from build123d import *

# Parameters (mm, degrees)
SKETCH1_R                = 2.5
BOSS_EXTRUDE1_DEPTH      = 4
CONVERT_SOLID1_OUTLINE_R = 2.5
CONVERT_SOLID1_DEPTH     = 2.5
EDGE_FLANGE1_DEPTH       = 20
EDGE_FLANGE1_BEND_DEPTH  = 20
EDGE_FLANGE2_DEPTH       = 20
EDGE_FLANGE2_BEND_DEPTH  = 20
SKETCH14_R               = 2.5
CUT_EXTRUDE1_DEPTH       = 4


# Read off the part's stored shape, not the designer's step: Convert-Solid1
# Sheet-metal steps are written as plain solids
with BuildPart() as part:
    # Sketch1 → Boss-Extrude1 (new body)
    with BuildSketch(Plane.XY):
        with BuildLine():
            Line((-474.195090562, 127.525252525), (-477.445756062, 127.525252525))
            ThreePointArc((-477.445756062, 127.525252525), (-484.91471638, 109.01150893), (-490.83715139, 89.946650322))
            Line((-490.83715139, 89.946650322), (-520.264617773, 89.946650322))
            Line((-520.264617773, 89.946650322), (-520.264617773, 69.946650322))
            Line((-520.264617773, 69.946650322), (-495.264617773, 69.946650322))
            ThreePointArc((-495.264617773, 69.946650322), (-499, 27.525252525), (-495.264617773, -14.896145272))
            Line((-495.264617773, -14.896145272), (-520.264617773, -14.896145272))
            Line((-520.264617773, -14.896145272), (-520.264617773, -34.896145272))
            Line((-520.264617773, -34.896145272), (-490.83715139, -34.896145272))
            ThreePointArc((-490.83715139, -34.896145272), (-484.91471638, -53.961003879), (-477.445756062, -72.474747475))
            Line((-477.445756062, -72.474747475), (-474.195090562, -72.474747475))
            ThreePointArc((-474.195090562, -72.474747475), (-470.012418883, -70.21432), (-469.611597595, -65.476850524))
            ThreePointArc((-469.611597595, -65.476850524), (-489, 27.525252525), (-469.611597595, 120.527355575))
            ThreePointArc((-469.611597595, 120.527355575), (-470.012418883, 125.264825051), (-474.195090562, 127.525252525))
        make_face()
        with Locations(Location((-488.148813177, 79.946650322, 0), (0, 0, 180))):
            Circle(SKETCH1_R, mode=Mode.SUBTRACT)
        with Locations((-494, 27.525252525)):
            Circle(SKETCH1_R, mode=Mode.SUBTRACT)
        with Locations((-488.148813177, -24.896145272)):
            Circle(SKETCH1_R, mode=Mode.SUBTRACT)
        with Locations((-476.297445473, -62.474747475)):
            Circle(SKETCH1_R, mode=Mode.SUBTRACT)
        with Locations(Location((-476.297445473, 117.525252525, 0), (0, 0, 180))):
            Circle(SKETCH1_R, mode=Mode.SUBTRACT)
    extrude(amount=BOSS_EXTRUDE1_DEPTH)

    # Convert-Solid1 outline → Convert-Solid1 (cut)
    with BuildSketch(Plane.XY):
        with BuildLine():
            ThreePointArc((-490.83715139, -34.896145272), (-484.91471638, -53.961003879), (-477.445756062, -72.474747475))
            Line((-477.445756062, -72.474747475), (-474.195090562, -72.474747475))
            ThreePointArc((-474.195090562, -72.474747475), (-470.012418883, -70.21432), (-469.611597595, -65.476850524))
            ThreePointArc((-469.611597595, -65.476850524), (-489, 27.525252525), (-469.611597595, 120.527355575))
            ThreePointArc((-469.611597595, 120.527355575), (-470.012418883, 125.264825051), (-474.195090562, 127.525252525))
            Line((-474.195090562, 127.525252525), (-477.445756062, 127.525252525))
            ThreePointArc((-477.445756062, 127.525252525), (-484.91471638, 109.011508929), (-490.83715139, 89.946650322))
            Line((-490.83715139, 89.946650322), (-520.264617773, 89.946650322))
            Line((-520.264617773, 89.946650322), (-520.264617773, 69.946650322))
            Line((-520.264617773, 69.946650322), (-495.264617773, 69.946650322))
            ThreePointArc((-495.264617773, 69.946650322), (-499, 27.525252525), (-495.264617773, -14.896145272))
            Line((-495.264617773, -14.896145272), (-520.264617773, -14.896145272))
            Line((-520.264617773, -14.896145272), (-520.264617773, -34.896145272))
            Line((-520.264617773, -34.896145272), (-490.83715139, -34.896145272))
        make_face()
        with Locations((-488.148813177, -24.896145272)):
            Circle(CONVERT_SOLID1_OUTLINE_R, mode=Mode.SUBTRACT)
        with Locations((-476.297445473, -62.474747475)):
            Circle(CONVERT_SOLID1_OUTLINE_R, mode=Mode.SUBTRACT)
        with Locations((-494, 27.525252525)):
            Circle(CONVERT_SOLID1_OUTLINE_R, mode=Mode.SUBTRACT)
        with Locations((-488.148813177, 79.946650322)):
            Circle(CONVERT_SOLID1_OUTLINE_R, mode=Mode.SUBTRACT)
        with Locations((-476.297445473, 117.525252525)):
            Circle(CONVERT_SOLID1_OUTLINE_R, mode=Mode.SUBTRACT)
    extrude(amount=CONVERT_SOLID1_DEPTH, mode=Mode.SUBTRACT)

    # Edge-Flange1 section (across the edge) → Edge-Flange1 (add)
    with BuildSketch(Plane(origin=(-521.264617773, 89.946650322, 4), x_dir=(1, 0, 0), z_dir=(0, -1, 0))):
        with BuildLine():
            Line((-1.5, 1), (-1.5, 8.5))
            Line((-1.5, 8.5), (0, 8.5))
            Line((0, 8.5), (0, 1))
            ThreePointArc((0, 1), (0.292893219, 0.292893219), (1, 0))
            Line((1, 0), (1, -1.5))
            ThreePointArc((1, -1.5), (-0.767766953, -0.767766953), (-1.5, 1))
        make_face()
    extrude(amount=EDGE_FLANGE1_DEPTH)

    # Edge-Flange1 section 2 (across the edge) → Edge-Flange1 bend (add)
    with BuildSketch(Plane(origin=(-521.264617773, -14.896145272, 4), x_dir=(1, 0, 0), z_dir=(0, -1, 0))):
        with BuildLine():
            Line((-1.5, 1), (-1.5, 8.5))
            Line((-1.5, 8.5), (0, 8.5))
            Line((0, 8.5), (0, 1))
            ThreePointArc((0, 1), (0.292893219, 0.292893219), (1, 0))
            Line((1, 0), (1, -1.5))
            ThreePointArc((1, -1.5), (-0.767766953, -0.767766953), (-1.5, 1))
        make_face()
    extrude(amount=EDGE_FLANGE1_BEND_DEPTH)

    # Edge-Flange2 section (across the edge) → Edge-Flange2 (add)
    with BuildSketch(Plane(origin=(-522.764617773, 69.946650322, 13.5), x_dir=(0, 0, -1), z_dir=(0, 1, 0))):
        with BuildLine():
            Line((-1.5, 1), (-1.5, 18.5))
            Line((-1.5, 18.5), (0, 18.5))
            Line((0, 18.5), (0, 1))
            ThreePointArc((0, 1), (0.292893219, 0.292893219), (1, 0))
            Line((1, 0), (1, -1.5))
            ThreePointArc((1, -1.5), (-0.767766953, -0.767766953), (-1.5, 1))
        make_face()
    extrude(amount=EDGE_FLANGE2_DEPTH)

    # Edge-Flange2 section 2 (across the edge) → Edge-Flange2 bend (add)
    with BuildSketch(Plane(origin=(-522.764617773, -34.896145272, 13.5), x_dir=(0, 0, -1), z_dir=(0, 1, 0))):
        with BuildLine():
            Line((-1.5, 1), (-1.5, 18.5))
            Line((-1.5, 18.5), (0, 18.5))
            Line((0, 18.5), (0, 1))
            ThreePointArc((0, 1), (0.292893219, 0.292893219), (1, 0))
            Line((1, 0), (1, -1.5))
            ThreePointArc((1, -1.5), (-0.767766953, -0.767766953), (-1.5, 1))
        make_face()
    extrude(amount=EDGE_FLANGE2_BEND_DEPTH)

    # Sketch14 → Cut-Extrude1 (cut)
    with BuildSketch(Plane.XY.offset(15)):
        with Locations((-534.014617773, 74.799905576)):
            Circle(SKETCH14_R)
        with Locations((-534.014617773, -20.042890014)):
            Circle(SKETCH14_R)
        with Locations((-534.014617773, -30.042890014)):
            Circle(SKETCH14_R)
        with Locations((-534.014617773, 84.799905576)):
            Circle(SKETCH14_R)
    extrude(amount=-CUT_EXTRUDE1_DEPTH, mode=Mode.SUBTRACT)


solid = part.part
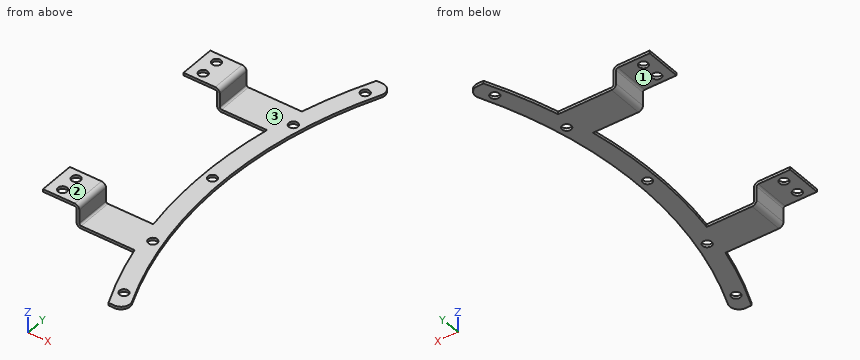
CAD build for the part. Positions are in the model's coordinates, mm. Face numbers are marked on the shaded views. A direction names the side the tool comes from. Round coordinates to 2 decimals unless told otherwise and drop trailing zeros. Loops run counter-clockwise (first coordinate to the right, second up) from the corner with the lowest first, then second, coordinate; pieces in that order, holes last.
(1) Drop flat-ended pins along their axis: pin 1 (8 mm diameter, centred on x = -532.5, y = -29, fed in from -Z); pin 2 (2 mm diameter, centred on y = 82, z = 9.5, fed in from +X); pin 3 (4 mm diameter, centred on x = -523.5, z = 8.5, fed in from +Y). Give the stop position or say it passes through.
(2) Cut at B-B (x = -518). Give the cut face in (y, z), plus the area to 3 significant figures.
(3) Wall check: line 1 along Z through (x, y) = (-518, 83.5); line 2 along Y through (x, z) = (-493, 3.5); line 3 along X through (y, z) = (107, 3.5). Give the ranges that are in metal, low to high.
(4) Which spindle directions (+Z, -Z, +X, -X, +Y, -Y) get a long thin tool onto all of the face, cutting with end or side? Do the marked faces 1, 2 and 3. Say none if no direction does.
(5) Cut at A-A (z = 9.25). Give the cut face in (x, y), plus the area to 3 significant figures.
Findings below:
1. pin 1: stops at z = 13.5
1. pin 2: stops at x = -521.26
1. pin 3: stops at y = 89.95
2. outline: (-34.9, 2.5) - (-14.9, 2.5) - (-14.9, 4) - (-34.9, 4) - close; (69.95, 2.5) - (89.95, 2.5) - (89.95, 4) - (69.95, 4) - close
2. area: 60.0 mm2
3. line 1: z = 2.5 to 4
3. line 2: y = -34.9 to 25.23, 29.82 to 89.95
3. line 3: x = -485.62 to -475.01
4. face 1: -Z, -X, +Y, -Y
4. face 2: +Z, +X, -X, +Y, -Y
4. face 3: +Z, +X, +Y, -Y
5. outline: (-522.76, -34.9) - (-521.26, -34.9) - (-521.26, -14.9) - (-522.76, -14.9) - close; (-522.76, 69.95) - (-521.26, 69.95) - (-521.26, 89.95) - (-522.76, 89.95) - close
5. area: 60.0 mm2
